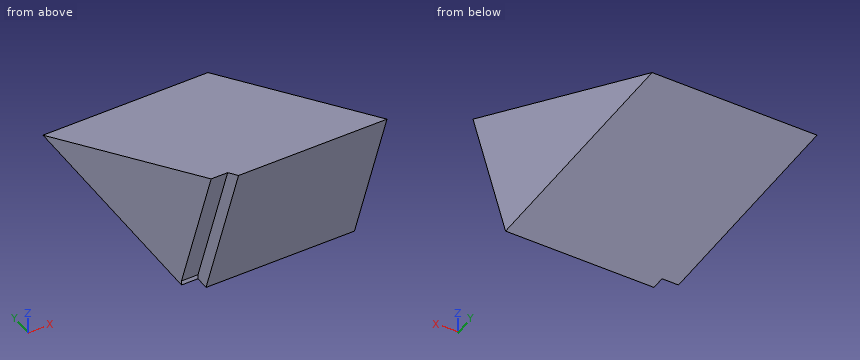
from build123d import *

# Parameters (mm, degrees)
F0_W     = 30
F0_H     = 10
F1_DEPTH = 30
F3_DEPTH = 30.001
F4_W     = 3
F4_H     = 31.6227766017
F5_DEPTH = 2.6
F7_DEPTH = 3


with BuildPart() as f1:
    # F0 (on Top) → F1 (new body)
    with BuildSketch(Plane.XY):
        Polygon((15, 22.5), (-15, 22.5), (-15, -19.5), (-15, -22.5), (15, -22.5), align=None)
        with Locations((0, -27.5)):
            Rectangle(F0_W, F0_H)
    extrude(amount=F1_DEPTH)

    # F2 (on face) → F3 (cut, through all)
    with BuildSketch(Plane.YZ.offset(15)):
        Polygon((-32.5, 0), (-22.5, 0), (-32.5, 30), align=None)
        Polygon((22.5, 30), (-32.5, 30), (22.5, 0), align=None)
    extrude(amount=-F3_DEPTH, mode=Mode.SUBTRACT)

    # F4 (on face) → F5 (cut)
    with BuildSketch(Plane(origin=(0, -20.25, -6.75), x_dir=(1, 0, 0), z_dir=(0, -0.9486832981, -0.316227766))):
        with Locations((-13.5, 22.9265130362)):
            Rectangle(F4_W, F4_H)
    extrude(amount=-F5_DEPTH, mode=Mode.SUBTRACT)

    # F6 (on face) → F7 (cut)
    with BuildSketch(Plane(origin=(-15, 0, 0), x_dir=(0, -1, 0), z_dir=(-1, 0, 0))):
        Polygon((22.5, 0), (20.0334234251, 0.8221921916), (20.0334234251, 0), align=None)
    extrude(amount=-F7_DEPTH, mode=Mode.SUBTRACT)


solid = f1.part
The listing builds one solid part. Answer for the finished solid, in the listing's coordinates (mm). Round coordinates to 2 decimals unless told otherwise and drop trailing zeros. Loops run counter-clockwise (first coordinate to the right, second up) from the corner with the lowest first, then second, coordinate; pieces in that order, holes last. Notation, with made-up numbers: M -39,-8.5 L 16,-8.5 A26 cw 16,11.5 Z; hole C -32,75 d3. An arc over 180 degrees is marked long. Return JSON: item names as keys, results as strings.
Q1. Find section C-C, the plane x = 8.75. Determine the outline of the cut face in (y, z), plus the area to 3 significant figures.
Results list:
{"outline": "M -32.5,30 L -22.5,0 L 22.5,0 Z", "area": "675 mm2"}
Q2. Find the intervals of material crossed by line 1 along Z through (x, y) = (-11.75, -7); line 2 along Y through (x, z) = (10, 13); line 3 along Z through (x, y) = (12, -11), in increasing order. Write a range as from..to.
Results list:
{"line 1": "z = 0..16.09", "line 2": "y = -26.83..-1.33", "line 3": "z = 0..18.27"}
Q3. This flat-tipped pin is pushed along its axis until it touches: pin 1 Ø3 at (x, z) = (4, 20) entering from -Y. Where does it stop, or does it pass through?
Results list:
{"pin 1": "stops at y = -29.67"}
Q4. Find section D-D, the plane y = -26.5. Determine the outline of the cut face in (x, z).
Results list:
{"outline": "M -15,20.22 L -12,20.22 L -12,12 L 15,12 L 15,26.73 L -15,26.73 Z"}
Q5. Find section B-B, the plane z = 17.5. Determine the outline of the cut face in (x, y), plus the area to 3 significant figures.
Results list:
{"outline": "M -15,-25.59 L -12,-25.59 L -12,-28.33 L 15,-28.33 L 15,-9.58 L -15,-9.58 Z", "area": "554 mm2"}
Q6. Find section A-A, the plane y = 17. Determine the outline of the cut face in (x, z), plus the area to 3 significant figures.
Results list:
{"outline": "M -15,0 L 15,0 L 15,3 L -15,3 Z", "area": "90.0 mm2"}
